from build123d import *

# Parameters (mm, degrees)
ESBO_O1_R                = 1.5
ESBO_O1_R_2              = 5
ESBO_O1_R_3              = 2
RESSALTO_EXTRUS_O1_DEPTH = 3


with BuildPart() as part:
    # Esboço1 → Ressalto-extrusão1 (new body)
    with BuildSketch(Plane.XY):
        with BuildLine():
            Line((95, -40), (-95, -40))
            ThreePointArc((-95, -40), (-98.535533906, -38.535533906), (-100, -35))
            Line((-100, -35), (-100, 35))
            ThreePointArc((-100, 35), (-98.535533906, 38.535533906), (-95, 40))
            Line((-95, 40), (95, 40))
            ThreePointArc((95, 40), (98.535533906, 38.535533906), (100, 35))
            Line((100, 35), (100, -35))
            ThreePointArc((100, -35), (98.535533906, -38.535533906), (95, -40))
        make_face()
        with Locations((-90, 30)):
            Circle(ESBO_O1_R, mode=Mode.SUBTRACT)
        with Locations((90, 30)):
            Circle(ESBO_O1_R, mode=Mode.SUBTRACT)
        with Locations((90, -30)):
            Circle(ESBO_O1_R, mode=Mode.SUBTRACT)
        with Locations((-90, -30)):
            Circle(ESBO_O1_R, mode=Mode.SUBTRACT)
        with Locations((-85, 0)):
            Circle(ESBO_O1_R_2, mode=Mode.SUBTRACT)
        with Locations((85, 0)):
            Circle(ESBO_O1_R_2, mode=Mode.SUBTRACT)
        with Locations((93, 6.67)):
            Circle(ESBO_O1_R_3, mode=Mode.SUBTRACT)
        with Locations((93, -6.67)):
            Circle(ESBO_O1_R_3, mode=Mode.SUBTRACT)
        with Locations(Location((77, -6.67, 0), (0, 0, 180))):
            Circle(ESBO_O1_R_3, mode=Mode.SUBTRACT)
        with Locations(Location((77, 6.67, 0), (0, 0, 180))):
            Circle(ESBO_O1_R_3, mode=Mode.SUBTRACT)
        with Locations((-77, -6.67)):
            Circle(ESBO_O1_R_3, mode=Mode.SUBTRACT)
        with Locations(Location((-93, -6.67, 0), (0, 0, 180))):
            Circle(ESBO_O1_R_3, mode=Mode.SUBTRACT)
        with Locations(Location((-93, 6.67, 0), (0, 0, 180))):
            Circle(ESBO_O1_R_3, mode=Mode.SUBTRACT)
        with Locations((-77, 6.67)):
            Circle(ESBO_O1_R_3, mode=Mode.SUBTRACT)
    extrude(amount=RESSALTO_EXTRUS_O1_DEPTH)


solid = part.part
Input: part model. Units: mm. Frame: model coordinates. Coordinates: 2 decimals unless noted, no trailing zeros. Loops run counter-clockwise (first coordinate to the right, second up) from the corner with the lowest first, then second, coordinate; pieces in that order, holes last. Notation, with made-up numbers: (4.25, -36.5) -> (60.25, -36.5) arc R15 cw to (60.25, -29.5) -> close; hole circle Ø4 at (-29.5, 46). An arc over 180 degrees is marked (long way). Write item = value, one per line. Start each with the question number.
Item 1: Material intervals for line 1 (Y direction, x = -93, z = 1.35); line 2 (Y direction, x = 85, z = 1.4); line 3 (Y direction, x = -80.5, z = 2.95), sorted ascending.
Item 2: Cut plane A-A, the plane x = -85. Return loops of the section in (y, z).
Item 3: First-contact query: P1, Ø3.5, axis at x = 77, y = -6.67, coming from the -Z side. Flat tip, straight axial feed; report the tip coordinate or a pass-through.
Item 4: Cut plane B-B, the plane x = 77. Return loops of the section in (y, z), plus the area to 3 significant figures.
Item 5: Cut plane C-C, the plane z = 0.55. Count the separate pieces of the cut face and the enclosed holes in it, plus the area to 3 significant figures.
Item 6: Mould query, pull axis Y, two halves, no side actions, for faces 1 (the face through (-75.092, -6.069, 1.479)), 2 (the face through (-98, -39, 1)), 3 (the face through (1, 1, 3)). Classes: pulls with the +Y half, pulls with the -Y half, needs draft (parallel to the pull), parting line crosses it, or undercut.
Ans:
q1.line_1 = -40 to -8.67, -4.67 to 4.67, 8.67 to 40
q1.line_2 = -40 to -5, 5 to 40
q1.line_3 = -40 to -2.18, 2.18 to 40
q2.outline = (-40, 0) -> (-5, 0) -> (-5, 3) -> (-40, 3) -> close; (5, 0) -> (40, 0) -> (40, 3) -> (5, 3) -> close
q3.P1 = through
q4.outline = (-40, 0) -> (-8.67, 0) -> (-8.67, 3) -> (-40, 3) -> close; (-4.67, 0) -> (4.67, 0) -> (4.67, 3) -> (-4.67, 3) -> close; (8.67, 0) -> (40, 0) -> (40, 3) -> (8.67, 3) -> close
q4.area = 216 mm²
q5.separate_pieces = 1
q5.enclosed_holes = 14
q5.area = 15,700 mm²
q6.face_1 = undercut
q6.face_2 = pulls with the -Y half
q6.face_3 = needs draft
